For this review, take the finished solid that the model builds, in its own axes (mm). A direction names the side the tool comes from. Give positions to 0.01 mm unless a question says otherwise; leave off trailing zeros. Loops run counter-clockwise (first coordinate to the right, second up) from the corner with the lowest first, then second, coordinate; pieces in that order, holes last. Notation, with made-up numbers: (57.25, 12.5) -> (61.25, 12.5) arc R24 ccw to (61.25, 26.5) -> close; hole circle Ø9 at (-40, 59). An arc over 180 degrees is marked (long way). One line per question, with ' | ' between items. Start each with the question number.
(1) Consider section A-A (x = 35). Write out the cut boundary in (y, z).
(2) Consider section C-C (z = 50.5). Write out the cut boundary in (x, y), and give its area (4 significant figures).
(3) Tool access review of faces 1 (the flat face through (35, 20, 55)), 2 (the flat face through (45, 22, 32)): name each direction out of +Z, -Z, +X, -X, +Y, -Y from which nothing blocks a thin tool from reaching the whole face with its end or side.
(4) Consider section B-B (y = 6). Write out the cut boundary in (x, z), and give its area (4 significant figures).
(5) Wall thickness on probe 1 along Y at (x, z) = (30, 52); probe 2 along X at (y, z) = (18, 62.5); probe 3 along Z at (x, y) = (27, 2): over which ranges is each line inside the solid? List them lowest first.
(6) Consider section D-D (x = 13). Write out the cut boundary in (y, z).
(7) Insertion check: P1, Ø4, axis at x = 37, y = 9.5, coming from the +Z side; P2, Ø6, axis at x = 34.5, z = 52, coming from the -Y side; P3, Ø10, axis at y = 6, z = 52, coming from the +X side. Each pin has a flat end and moves straight along its axis. Give the tip position at first contact, or say it passes through.
from build123d import *

# Parameters (mm, degrees)
F0_W     = 45
F0_H     = 45
F1_DEPTH = 65
F2_W     = 20
F2_H     = 20
F3_DEPTH = 20
F4_SIZE  = 10


with BuildPart() as f1:
    # F0 (on Top) → F1 (new body)
    with BuildSketch(Plane.XY):
        with Locations((22.5, 22.5)):
            Rectangle(F0_W, F0_H)
    extrude(amount=F1_DEPTH)

    # F2 (on face) → F3 (cut)
    with BuildSketch(Plane.YZ.offset(45)):
        with Locations((10, 55)):
            Rectangle(F2_W, F2_H)
    extrude(amount=-F3_DEPTH, mode=Mode.SUBTRACT)

    # F4
    f4_edges = [f1.edges().sort_by_distance(p)[0] for p in [
        (22.5, 45, 0),
    ]]
    chamfer(f4_edges, length=F4_SIZE)


solid = f1.part
A:
1) outline: (0, 0) -> (35, 0) -> (45, 10) -> (45, 65) -> (20, 65) -> (20, 45) -> (0, 45) -> close
2) outline: (0, 0) -> (25, 0) -> (25, 20) -> (45, 20) -> (45, 45) -> (0, 45) -> close | area: 1,625 mm^2
3) face 1: +Z, +X, -Y | face 2: +Z, -Z, +X, +Y, -Y
4) outline: (0, 0) -> (45, 0) -> (45, 45) -> (25, 45) -> (25, 65) -> (0, 65) -> close | area: 2,525 mm^2
5) probe 1: y = 20 to 45 | probe 2: x = 0 to 25 | probe 3: z = 0 to 45
6) outline: (0, 0) -> (35, 0) -> (45, 10) -> (45, 65) -> (0, 65) -> close
7) P1: stops at z = 45 | P2: stops at y = 20 | P3: stops at x = 25
